Geometry check sheet. Reference: the model listing, model coordinates, mm. A direction names the side the tool comes from. Coordinates: 2 decimals unless noted, no trailing zeros. Order: outer loops, then holes, each group sorted by start corner. A loop starts at its lowest first (then second) coordinate and runs counter-clockwise, first axis right, second up. Notation, with made-up numbers: (66.5, 1) -> (123.5, 1) arc R22 ccw to (123.5, 38) -> close; hole circle Ø3 at (53.25, -29). An arc over 180 degrees is marked (long way). Answer in a Markdown table with one row per item. Add a question column.
```python
from build123d import *

# Parameters (mm, degrees)
EXTRUDE1_DEPTH        = 5
SKETCH3_R             = 1.4732
CUT_EXTRUDE2_DEPTH    = 6
SKETCH4_W             = 12
SKETCH4_H             = 10
EXTRUDE2_DEPTH        = 10
FILLET1_R             = 4
CUT_EXTRUDE3_DEPTH    = 39
F_8_CLEARANCE_HOLE1_D = 4.3053


with BuildPart() as part:
    # Sketch1 → Extrude1 (new body)
    with BuildSketch(Plane.XY):
        Polygon((0, 39), (0, -39), (12, -39), (12, 0), (12, 39), align=None)
    extrude(amount=EXTRUDE1_DEPTH)

    # Sketch3 → Cut-Extrude2 (cut, through all)
    with BuildSketch(Plane.XY.offset(5)):
        with Locations((6, 3)):
            Circle(SKETCH3_R)
    extrude(amount=-CUT_EXTRUDE2_DEPTH, mode=Mode.SUBTRACT)

    # Sketch4 → Extrude2 (add)
    with BuildSketch(Plane(origin=(0, 0, 0), x_dir=(-1, 0, 0), z_dir=(0, 0, -1))):
        with Locations((-6, 34)):
            Rectangle(SKETCH4_W, SKETCH4_H)
        with Locations((-6, -34)):
            Rectangle(SKETCH4_W, SKETCH4_H)
    extrude(amount=EXTRUDE2_DEPTH)

    # Fillet1
    fillet1_edges = [part.edges().sort_by_distance(p)[0] for p in [
        (6, -29, 0),
        (6, 29, 0),
    ]]
    fillet(fillet1_edges, radius=FILLET1_R)

    # Sketch5 → Cut-Extrude3 (cut)
    with BuildSketch(Plane(origin=(0, 0, 0), x_dir=(1, 0, 0), z_dir=(0, 1, 0))):
        Polygon((0, 10), (0, 6.192), (12, 2.931672159), (12, 8.784609691), (12, 10), align=None)
    extrude(amount=-CUT_EXTRUDE3_DEPTH, mode=Mode.SUBTRACT)

    # #8 Clearance Hole1 (through all)
    with Locations(Plane(origin=(6, 34, 5), x_dir=(1, 0, 0), z_dir=(0, 0, 1))):
        with Locations((0, 0), (0, -68)):
            Hole(F_8_CLEARANCE_HOLE1_D / 2)


solid = part.part
```
(1) Mould release check, pull along X, two halves, no side actions. Record for faces 3 (the face through (3.947, 34.647, -2.605)), 4 (the face through (5.916, -31.602, -4.585)), 5 (the face through (6, -39, 1)), 6 (the face through (3.947, -33.353, -0.144)): +X half, -X half, draft (parallel to the pull), parting line (faces both ways), or undercut.
(2) Cross-section at D-D (y = 3). Enter the section's corners in (x, z), plus the area to 3 significant figures.
(3) Scan lines: line 1 along Y through (x, z) = (6, -4.75); line 2 along Y through (x, z) = (6, 1.6); line 3 along Y through (x, z) = (6.75, 1.5). Record each from-to range of solid material in increasing order.
(4) Go/stop test with a flat-tipped pin: P1, Ø5, axis at x = 6, z = -8, coming from the -Y side. Record where the tip stops, or that it passes through.
(5) Cross-section at B-B (z = -8.5). Enter the section's corners in (x, y), plus the area to 3 significant figures.
(6) Cross-section at C-C (x = 6). Enter the section's corners in (y, z), plus the area to 3 significant figures.
(7) Access from +Z, -Z, +X, -X, +Y, -Y to the whole of each face (thin tool, end or side, straight path). Record for faces 1 (the face through (6, 39, -2)), 2 (the face through (2, -29, -5)).
(8) Cross-section at A-A (y = 34). Enter the section's corners in (x, z).
Checks:
| question | item | result |
|---|---|---|
| 1 | face 3 | undercut |
| 1 | face 4 | +X half |
| 1 | face 5 | draft |
| 1 | face 6 | undercut |
| 2 | outline | (0, 0) -> (4.53, 0) -> (4.53, 5) -> (0, 5) -> close; (7.47, 0) -> (12, 0) -> (12, 5) -> (7.47, 5) -> close |
| 2 | area | 45.3 mm² |
| 3 | line 1 | 29 to 31.85, 36.15 to 39 |
| 3 | line 2 | -39 to -36.15, -31.85 to 1.53, 4.47 to 31.85, 36.15 to 39 |
| 3 | line 3 | -39 to -36.02, -31.98 to 1.73, 4.27 to 31.98, 36.02 to 39 |
| 4 | P1 | y = 29 |
| 5 | outline | (0, 29) -> (12, 29) -> (12, 39) -> (0, 39) -> close; hole circle Ø4.31 at (6, 34) |
| 5 | area | 105 mm² |
| 6 | outline | (-39, -4.56) -> (-36.15, -4.56) -> (-36.15, 5) -> (-39, 5) -> close; (-31.85, -4.56) -> (-29, -4.56) -> (-29, -4) arc R4 cw to (-25, 0) -> (1.53, 0) -> (1.53, 5) -> (-31.85, 5) -> close; (4.47, 0) -> (25, 0) arc R4 cw to (29, -4) -> (29, -10) -> (31.85, -10) -> (31.85, 5) -> (4.47, 5) -> close; (36.15, -10) -> (39, -10) -> (39, 5) -> (36.15, 5) -> close |
| 6 | area | 422 mm² |
| 7 | face 1 | +Z, -Z, +X, -X, +Y |
| 7 | face 2 | -Z, +X, -X |
| 8 | outline | (0, -10) -> (3.85, -10) -> (3.85, 5) -> (0, 5) -> close; (8.15, -10) -> (12, -10) -> (12, 5) -> (8.15, 5) -> close |
